CAD build for the part. Positions are in the model's coordinates, mm. A direction names the side the tool comes from. Round coordinates to 2 decimals unless told otherwise and drop trailing zeros. Write each loop counter-clockwise with the first axis right and the second up, starting at its lowest first coordinate (ties: lowest second). Pieces come first, ordered by that corner, then holes. Notation, with made-up numbers: (-39.75, 13) -> (-5.75, 13) arc R14 cw to (-5.75, 30) -> close; hole circle Ø7 at (-6.5, -18). An arc over 180 degrees is marked (long way). Put each result on its own line as item: value. Start each with the question number.
1. Saw through at D-D on x = 45.5. List the corners of the cut face in (y, z).
2. Pull direction Y, two halves, no side cores. Call faces 1 (the cylindrical face through (52.31, -4.93, -0.96)), 2 (the cylindrical face through (55.453, -4.93, 0.716)), 3 (the flat face through (-1, -7, 0)), 4 (the flat face through (-1, -10, 0)): pulls with the +Y half, pulls with the -Y half, needs draft (parallel to the pull), parting line crosses it, or undercut.
3. Saw through at C-C on y = -5. List the corners of the cut face in (x, z), and give its area (3 significant figures).
4. Saw through at A-A on x = 24.5. List the corners of the cut face in (y, z), and give its area (3 significant figures).
5. Flat gauge pins, fed straight in: P1, Ø3, axis at x = 50, z = 0, coming from the -Y side; P2, Ø1, axis at y = -2, z = -1, coming from the -X side. Where does each tip first touch, or does it go through?
6. Saw through at B-B on z = 0. List the corners of the cut face in (x, y).
7. 3-axis set-ups, long thin cutter, end or side, ignore diameter. For faces 5 (the flat face through (-1, -1, -5.5)), 6 (the cylindrical face through (-55.453, -4.93, -0.716)): which of +Z, -Z, +X, -X, +Y, -Y reach the whole face in a straight line?
8. Drill centre lines: line 1 (Z direction, x = 50, y = -8); line 2 (Y direction, x = 10.5, z = -3.5); line 3 (X direction, y = -1.75, z = 1.25). Where is each one in solid material? Low to high. Write a range as from..to.
from build123d import *

# Parameters (mm, degrees)
F0_R     = 2.5
F1_DEPTH = 10
F2_T     = 3


# Not quite as in the source:
# - a shell that OpenCascade refuses in one call is made with other operations: the cavity is built on its own and cut out


with BuildPart() as f1:
    # F0 (on Front) → F1 (new body)
    with BuildSketch(Plane.XZ):
        with BuildLine():
            Line((0, 5.5), (-50, 5.5))
            ThreePointArc((-50, 5.5), (-55.5, 0), (-50, -5.5))
            Line((-50, -5.5), (0, -5.5))
            Line((0, -5.5), (50, -5.5))
            ThreePointArc((50, -5.5), (55.5, 0), (50, 5.5))
            Line((50, 5.5), (0, 5.5))
        make_face()
        with Locations((-50, 0)):
            Circle(F0_R, mode=Mode.SUBTRACT)
        with Locations((50, 0)):
            Circle(F0_R, mode=Mode.SUBTRACT)
    extrude(amount=F1_DEPTH)

    # F2: shell of thickness 3, made by hand


with BuildPart() as f2_core1:
    # F2_t2: copy of F1
    add(f1.part)

    # the walls: a layer under each face that stays
    f2_faces = [f2_core1.faces().sort_by_distance(p)[0] for p in [
        (0, -10, 0),
        (47.5, -5, 0),
        (-52.5, -5, 0),
        (55.5, -5, 0),
        (0, 0, 0),
        (-55.5, -5, 0),
    ]]
    thicken(f2_faces, amount=-F2_T, mode=Mode.SUBTRACT)


with BuildPart() as f1_1:
    add(f1.part)

    # what is left inside the walls is the cavity
    f2_cavity = [f2_core1.part.solids().sort_by_distance(p)[0] for p in [
        (0, -3.03, -1.833333),
    ]]
    add(f2_cavity, mode=Mode.SUBTRACT)


solid = f1_1.part
Return value:
1. outline: (-10, -5.5) -> (-7, -5.5) -> (-7, -3.16) -> (-3, -3.16) -> (-3, -5.5) -> (0, -5.5) -> (0, 5.5) -> (-3, 5.5) -> (-3, 3.16) -> (-7, 3.16) -> (-7, 5.5) -> (-10, 5.5) -> close
2. face 1: needs draft
2. face 2: undercut
2. face 3: undercut
2. face 4: pulls with the -Y half
3. outline: circle Ø11 at (-50, 0); circle Ø11 at (50, 0); hole circle Ø5 at (-50, 0); hole circle Ø5 at (50, 0)
3. area: 151 mm^2
4. outline: (-10, -5.5) -> (-7, -5.5) -> (-7, 5.5) -> (-10, 5.5) -> close; (-3, -5.5) -> (0, -5.5) -> (0, 5.5) -> (-3, 5.5) -> close
4. area: 66.0 mm^2
5. P1: passes through
5. P2: stops at x = -55.48
6. outline: (-55.5, -10) -> (-52.5, -10) -> (-52.5, 0) -> (-55.5, 0) -> close; (-47.5, -10) -> (47.5, -10) -> (47.5, 0) -> (-47.5, 0) -> close; (52.5, -10) -> (55.5, -10) -> (55.5, 0) -> (52.5, 0) -> close; hole (-44.5, -7) -> (44.5, -7) -> (44.5, -3) -> (-44.5, -3) -> close
7. face 5: -Z, +X, -X, +Y, -Y
7. face 6: none
8. line 1: z = -5.5..-2.5, 2.5..5.5
8. line 2: y = -10..-7, -3..0
8. line 3: x = -55.36..-52.17, -47.83..47.83, 52.17..55.36
